```python
from build123d import *

# Parameters (mm, degrees)
BOSS_EXTRUDE3_START        = 15
SKETCH2_R                  = 12
BOSS_EXTRUDE3_DEPTH        = 15
F_13_0_13_DIAMETER_HOLE1_D = 13


with BuildPart() as part:
    # Sketch1 → Revolve1 (revolve)
    with BuildSketch(Plane.XY, mode=Mode.PRIVATE) as revolve1_sk:
        with BuildLine():
            Line((12, 0), (21, 0))
            Line((21, 0), (21, 60))
            Line((21, 60), (25, 60))
            Line((25, 60), (25, 69))
            Line((25, 69), (23, 69))
            ThreePointArc((23, 69), (19.845922252, 60.849571269), (12, 57))
            Line((12, 57), (12, 0))
        make_face()
    revolve(revolve1_sk.sketch.rotate(Axis((0, 0, 0), (0, 1, 0)), 90), axis=Axis((0, 0, 0), (0, 1, 0)))

    # Sketch2 → Boss-Extrude3 (add)
    with BuildSketch(Plane.XZ.offset(-60).offset(BOSS_EXTRUDE3_START)):
        with BuildLine():
            ThreePointArc((-60.125231169, 6.521519783), (-0.519935794, 36), (59.08535958, 6.521519783))
            ThreePointArc((59.08535958, 6.521519783), (60.308298463, 0), (59.08535958, -6.521519783))
            ThreePointArc((59.08535958, -6.521519783), (-0.519935794, -36), (-60.125231169, -6.521519783))
            ThreePointArc((-60.125231169, -6.521519783), (-61.348170052, 0), (-60.125231169, 6.521519783))
        make_face()
        with Locations(Location((0, 0, 0), (0, 0, 270))):
            Circle(SKETCH2_R, mode=Mode.SUBTRACT)
    extrude(amount=-BOSS_EXTRUDE3_DEPTH)

    # Ø13.0 (13) Diameter Hole1 (through all)
    with Locations(Plane(origin=(0, 60, 0), x_dir=(1, 0, 0), z_dir=(0, 1, 0))):
        with Locations((-42, 0), (42, 0)):
            Hole(F_13_0_13_DIAMETER_HOLE1_D / 2)

    # Sketch6 → Cut-Revolve5 (revolve, cut)
    with BuildSketch(Plane.XY, mode=Mode.PRIVATE) as cut_revolve5_sk:
        Polygon((21, 0), (12, 0), (12, 2.411542732), align=None)
    revolve(cut_revolve5_sk.sketch.rotate(Axis((0, 0, 0), (0, 1, 0)), 90), axis=Axis((0, 0, 0), (0, 1, 0)), mode=Mode.SUBTRACT)


solid = part.part
```
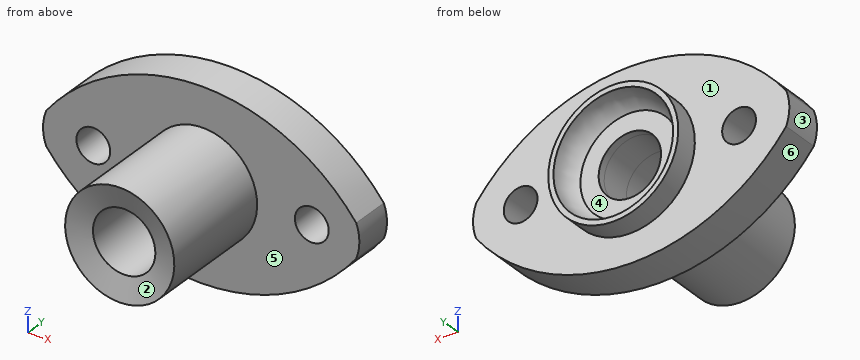
Read the model definition and answer for the solid it produces. Units are mm, in the model's axes. Face numbers are marked on the shaded views. A direction names the side the tool comes from. Give positions to 0.01 mm unless a question says otherwise; leave off trailing zeros. Order: outer loops, then holes, each group sorted by start corner. A loop starts at its lowest first (then second) coordinate and runs counter-clockwise, first axis right, second up.
(1) For the marked faces 4, 5 and 6, determine the directions among +Z, -Z, +X, -X, +Y, -Y from which every point of the face is accessible in a straight line to the end or side of a thin tool.
(2) Straight lines are drawn through the part: L1, parallel to Z at x = 0, y = 49.5; L2, parallel to X at y = 56, z = 5; L3, parallel to Y at x = -27, z = 10.5. For each, find the intervals that lie inside material, in ascending order.
(3) Find section B-B (x = 42). Give the vertices of the cut face in (y, z).
(4) Find section D-D (y = 6). Give the vertices of the cut face in (x, z), plus the area to 3 significant figures.
(5) Given pin 1 (8 mm diameter, centred on x = 42, z = 0, fed in from -Y); pin 2 (8 mm diameter, centred on y = 26.5, z = 12, fed in from -X); pin 3 (4 mm diameter, centred on x = -43, z = 5, fed in from +Y); pin 4 (3 mm diameter, centred on y = 13.5, z = -4.5, fed in from +X), each flat-ended and moving along its own axis, determine where each tip first touches the part or whether it passes through.
(6) Find section C-C (z = 0). Give the number of separate pieces and of enclosed holes in the cut face, plus the area to 3 significant figures.
(7) For a pull along X with two mould halves and no side action, classify the marked faces 1, 2 and 3 as released by +X, released by -X, zero draft, split by the parting line, or undercut.
(8) Find section A-A (y = 55). Give the vertices of the cut face in (x, z), plus the area to 3 significant figures.
Result sheet:
1. face 4: +Y
1. face 5: -Y
1. face 6: -Z, +Y, -Y
2. L1: z = -36 to -12, 12 to 36
2. L2: x = -60.64 to -46.15, -37.85 to -10.91, 10.91 to 37.85, 46.15 to 59.6
2. L3: y = 45 to 60
3. outline: (45, -22.78) - (60, -22.78) - (60, -6.5) - (45, -6.5) - close; (45, 6.5) - (60, 6.5) - (60, 22.78) - (45, 22.78) - close
4. outline: circle Ø42 at (0, 0); hole circle Ø24 at (0, 0)
4. area: 933 mm2
5. pin 1: passes through
5. pin 2: stops at x = -19.42
5. pin 3: stops at y = 60
5. pin 4: stops at x = 20.78
6. separate pieces: 4
6. enclosed holes: 0
6. area: 1,920 mm2
7. face 1: zero draft
7. face 2: undercut
7. face 3: released by -X
8. outline: (-60.13, -6.52) arc R75 ccw to (59.09, -6.52) arc R18 ccw to (59.09, 6.52) arc R75 ccw to (-60.13, 6.52) arc R18 ccw to start; hole circle Ø13 at (-42, 0); hole circle Ø24 at (0, 0); hole circle Ø13 at (42, 0)
8. area: 5,770 mm2
